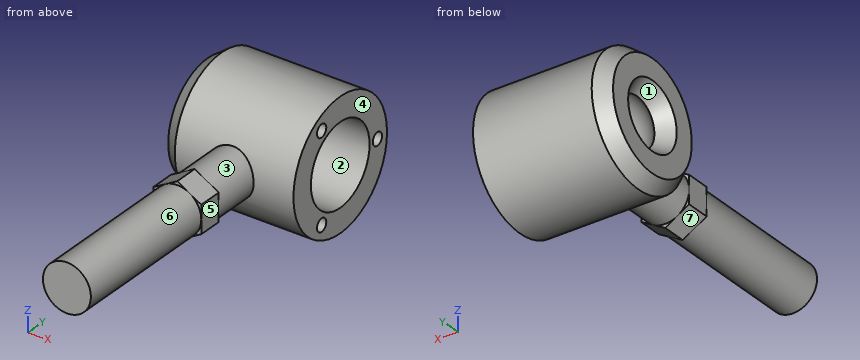
```python
from build123d import *

# Parameters (mm, degrees)
SKETCH2_R                            = 15
BOSS_EXTRUDE1_DEPTH                  = 30
BOSS_EXTRUDE1_DIRECTION_2_REACH      = 123.644
BOSS_EXTRUDE1_DIRECTION_2_END_RADIUS = 40.25
BOSS_EXTRUDE2_DEPTH                  = 15
BOSS_EXTRUDE3_START                  = 95
SKETCH4_R                            = 15
BOSS_EXTRUDE3_DEPTH                  = 95
SKETCH5_R                            = 4
CUT_EXTRUDE1_DEPTH                   = 20


with BuildPart() as part:
    # Sketch1 → Revolve1 (revolve)
    with BuildSketch(Plane.XY):
        with BuildLine():
            Line((8.523453836, 15), (-1.164911567, 20.895027572))
            Line((-1.164911567, 20.895027572), (-1.164911567, 33.880431222))
            Line((-1.164911567, 33.880431222), (7.573302349, 40.25))
            Line((7.573302349, 40.25), (81.835088433, 40.25))
            Line((81.835088433, 40.25), (81.835088433, 25.25))
            Line((81.835088433, 25.25), (28.835088433, 25.25))
            ThreePointArc((28.835088433, 25.25), (17.45940164, 22.542321309), (8.523453836, 15))
        make_face()
    revolve(axis=Axis((28.835088433, 0, 0), (-1, 0, 0)))

    # Sketch2 → Boss-Extrude1 (add)
    with BuildSketch(Plane(origin=(0, -40.25, 0), x_dir=(-1, 0, 0), z_dir=(0, -1, 0))):
        with Locations(Location((-41.897124258, 0, 0), (0, 0, 90))):
            Circle(SKETCH2_R)
    extrude(amount=BOSS_EXTRUDE1_DEPTH)

    # Boss-Extrude1 direction 2: up to this cylinder (the profile starts outside it)
    boss_extrude1_direction_2_end = Plane(origin=(41.897124, 0, 0), z_dir=(1, 0, 0)) * Cylinder(BOSS_EXTRUDE1_DIRECTION_2_END_RADIUS, 328.788, mode=Mode.PRIVATE)
    # Sketch2 → Boss-Extrude1 direction 2 (add, up to the surface)
    with BuildSketch(Plane(origin=(0, -40.25, 0), x_dir=(-1, 0, 0), z_dir=(0, -1, 0)), mode=Mode.PRIVATE) as boss_extrude1_direction_2_sk1:
        with Locations(Location((-41.897124258, 0, 0), (0, 0, 90))):
            Circle(SKETCH2_R)
    boss_extrude1_direction_2_tool1 = extrude(boss_extrude1_direction_2_sk1.sketch, amount=-BOSS_EXTRUDE1_DIRECTION_2_REACH, mode=Mode.PRIVATE) - boss_extrude1_direction_2_end
    add(boss_extrude1_direction_2_tool1.solids().sort_by_distance((41.897124, -40.25, 0))[0])
    add(boss_extrude1_direction_2_tool1.solids().sort_by_distance((41.897124, -40.25, 0))[1])

    # Sketch3 → Boss-Extrude2 (add)
    with BuildSketch(Plane.XZ.offset(70.25)):
        Polygon((56.897124258, -8.660254038), (56.897124258, 8.660254038), (41.897124258, 17.320508076), (26.897124258, 8.660254038), (26.897124258, -8.660254038), (41.897124258, -17.320508076), align=None)
    extrude(amount=BOSS_EXTRUDE2_DEPTH)

    # Sketch4 → Boss-Extrude3 (add)
    with BuildSketch(Plane.XZ.offset(85.25).offset(BOSS_EXTRUDE3_START)):
        with Locations(Location((41.897124258, 0, 0), (0, 0, 120))):
            Circle(SKETCH4_R)
    extrude(amount=-BOSS_EXTRUDE3_DEPTH)

    # Sketch5 → Cut-Extrude1 (cut)
    with BuildSketch(Plane(origin=(81.835088433, 0, 0), x_dir=(0, 0, -1), z_dir=(1, 0, 0))):
        with Locations(Location((0, 32, 0), (0, 0, 90))):
            Circle(SKETCH5_R)
        with Locations(Location((27.712812921, -16, 0), (0, 0, 90))):
            Circle(SKETCH5_R)
        with Locations(Location((-27.712812921, -16, 0), (0, 0, 90))):
            Circle(SKETCH5_R)
    extrude(amount=-CUT_EXTRUDE1_DEPTH, mode=Mode.SUBTRACT)


solid = part.part
```
Source: CAD feature listing. Evaluate the final solid. Frame: model axes, mm. Face numbers are marked on the shaded views. A direction names the side the tool comes from. Coordinates: 2 decimals unless noted, no trailing zeros. Write each loop counter-clockwise with the first axis right and the second up, starting at its lowest first coordinate (ties: lowest second). Pieces come first, ordered by that corner, then holes. Notation, with made-up numbers: M 18,41 L 39,41 A21 cw 39,52 Z; hole C 3,-6.75 d4. An arc over 180 degrees is marked long. Answer as a JSON object with one key per item and string values.
1. Contact query for flat-ended pins moving along their axis: P1, Ø4, axis at y = -15.5, z = -27.5, coming from the +X side; P2, Ø6, axis at y = 12.5, z = -4, coming from the +X side; P3, Ø3, axis at x = 37, z = 26.5, coming from the -Y side; P4, Ø12, axis at y = -44, z = -27, coming from the -X side. Output: stop coordinate, or through.
Evaluation:
{"P1": "x = 61.84", "P2": "x = 9.4", "P3": "y = -31.54", "P4": "through"}
2. Cut plane C-C on y = -148.5. Output: boundary loops of the cut face in (x, z), plus the area to 3 significant figures.
Evaluation:
{"outline": "C 41.9,0 d30", "area": "707 mm^2"}
3. Access query for the marked faces 5, 6 and 7. Directions: +Z, -Z, +X, -X, +Y, -Y. A direction counts if a zero-diameter tool reaches every point of the face in a straight line with its end or side. Return the directions, or none.
Evaluation:
{"face 5": "+Z, -Z, +X, -Y", "face 6": "-Y", "face 7": "-Z, -X, -Y"}
4. Ray query, L1, parallel to Z at x = 35.5, y = 1; L2, parallel to Z at x = 68, y = -16; L3, parallel to Y at x = 76, z = -1.5. Return the intervals inside material, ascending.
Evaluation:
{"L1": "-40.24 to -25.23, 25.23 to 40.24", "L2": "-36.93 to -31.71, -23.71 to -19.53, 19.53 to 23.71, 31.71 to 36.93", "L3": "-40.22 to -25.21, 25.21 to 28.29, 35.71 to 40.22"}
5. Draft query along Z for the marked faces 1, 2, 3 and 4. Return one class per face: released by +Z, released by -Z, zero draft, split by the parting line, or undercut.
Evaluation:
{"face 1": "undercut", "face 2": "undercut", "face 3": "split by the parting line", "face 4": "zero draft"}
6. Cut plane A-A on y = 0. Output: boundary loops of the cut face in (x, z).
Evaluation:
{"outline": "M -1.16,-33.88 L 7.57,-40.25 L 81.84,-40.25 L 81.84,-25.25 L 28.84,-25.25 A25.25 cw 8.52,-15 L -1.16,-20.9 Z; M -1.16,20.9 L 8.52,15 A25.25 cw 28.84,25.25 L 81.84,25.25 L 81.84,40.25 L 7.57,40.25 L -1.16,33.88 Z"}
7. Cut plane B-B on x = 64. Output: boundary loops of the cut face in (y, z).
Evaluation:
{"outline": "C 0,0 d80.5; hole C 0,0 d50.5; hole C -16,-27.71 d8; hole C -16,27.71 d8; hole C 32,0 d8"}
